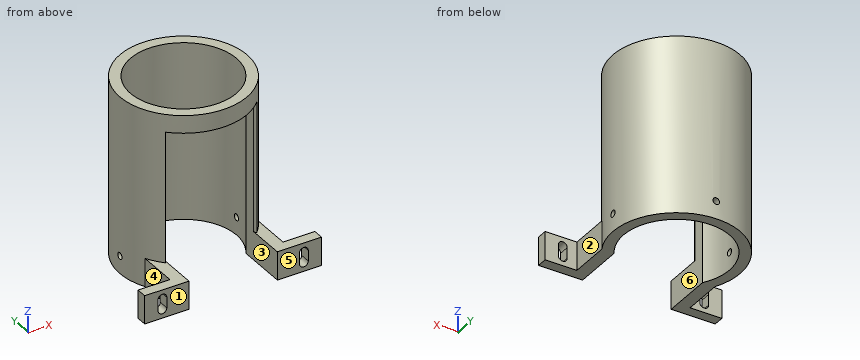
from build123d import *

# Parameters (mm, degrees)
SKETCH1_R                = 18
SKETCH1_R_2              = 15
BOSS_EXTRUDE1_DEPTH      = 50
SKETCH2_W                = 50
SKETCH2_H                = 8
BOSS_EXTRUDE2_DEPTH      = 3
BOSS_EXTRUDE5_REACH      = 69.315
BOSS_EXTRUDE5_END_RADIUS = 18
SKETCH9_W                = 32
SKETCH9_H                = 8
SKETCH4_W                = 37
SKETCH4_H                = 10
CUT_EXTRUDE1_DEPTH       = 75.204110398
CUT_EXTRUDE2_REACH       = 71.031
CUT_EXTRUDE2_END_RADIUS  = 15
SKETCH6_W                = 25
SKETCH6_H                = 45
FILLET1_R                = 1
CUT_EXTRUDE3_REACH       = 62.26
CUT_EXTRUDE3_END_RADIUS  = 18
SKETCH7_R                = 0.925
CIRPATTERN1_START        = 14.971451916
CIRPATTERN1_OUTLINE_R    = 0.925
CIRPATTERN1_DEPTH        = 3.028548184
CIRPATTERN1_START_2      = 14.9714519
CIRPATTERN1_2_OUTLINE_R  = 0.925
CIRPATTERN1_2_DEPTH      = 3.028548184


# Read off the part's stored shape, not the designer's step: CirPattern1
with BuildPart() as part:
    # Sketch1 → Boss-Extrude1 (new body)
    with BuildSketch(Plane.XY):
        Circle(SKETCH1_R)
        Circle(SKETCH1_R_2, mode=Mode.SUBTRACT)
    extrude(amount=BOSS_EXTRUDE1_DEPTH)



with BuildPart() as body_2:
    # Sketch2 → Boss-Extrude2 (new body)
    with BuildSketch(Plane(origin=(0, -22.5, 0), x_dir=(1, 0, 0), z_dir=(0, 1, 0))):
        with Locations((0, -4)):
            Rectangle(SKETCH2_W, SKETCH2_H)
        with BuildLine():
            Line((21.25, -2.5), (21.25, -5.5))
            ThreePointArc((21.25, -5.5), (20, -6.75), (18.75, -5.5))
            Line((18.75, -5.5), (18.75, -2.5))
            ThreePointArc((18.75, -2.5), (20, -1.25), (21.25, -2.5))
        make_face(mode=Mode.SUBTRACT)
        with BuildLine():
            Line((-21.25, -2.5), (-21.25, -5.5))
            ThreePointArc((-21.25, -5.5), (-20, -6.75), (-18.75, -5.5))
            Line((-18.75, -5.5), (-18.75, -2.5))
            ThreePointArc((-18.75, -2.5), (-20, -1.25), (-21.25, -2.5))
        make_face(mode=Mode.SUBTRACT)
    extrude(amount=BOSS_EXTRUDE2_DEPTH)


with BuildPart() as part_1:
    add(part.part)

    add(body_2.part)  # Boss-Extrude5 merges body 2
    # Boss-Extrude5: up to this cylinder (the profile starts outside it)
    boss_extrude5_end = Plane(origin=(0, 0, 4), z_dir=(0, 0, -1)) * Cylinder(BOSS_EXTRUDE5_END_RADIUS, 175.63, mode=Mode.PRIVATE)
    # Sketch9 → Boss-Extrude5 (add, up to the surface)
    with BuildSketch(Plane(origin=(0, -19.5, 0), x_dir=(1, 0, 0), z_dir=(0, 1, 0)), mode=Mode.PRIVATE) as boss_extrude5_sk1:
        with Locations((0, -4)):
            Rectangle(SKETCH9_W, SKETCH9_H)
    boss_extrude5_tool1 = extrude(boss_extrude5_sk1.sketch, amount=BOSS_EXTRUDE5_REACH, mode=Mode.PRIVATE) - boss_extrude5_end
    add(boss_extrude5_tool1.solids().sort_by_distance((0, -19.5, 4))[0])

    # Sketch4 → Cut-Extrude1 (cut, through all)
    with BuildSketch(Plane.ZY.offset(25)):
        with Locations((26.5, -17.5)):
            Rectangle(SKETCH4_W, SKETCH4_H)
    extrude(amount=-CUT_EXTRUDE1_DEPTH, mode=Mode.SUBTRACT)

    # Cut-Extrude2: up to this cylinder (the profile starts outside it)
    cut_extrude2_end = Plane(origin=(0, 0, 22.5), z_dir=(0, 0, -1)) * Cylinder(CUT_EXTRUDE2_END_RADIUS, 173.062, mode=Mode.PRIVATE)
    # Sketch6 → Cut-Extrude2 (cut, up to the surface)
    with BuildSketch(Plane.XZ.offset(22.5), mode=Mode.PRIVATE) as cut_extrude2_sk1:
        with Locations((0, 22.5)):
            Rectangle(SKETCH6_W, SKETCH6_H)
    cut_extrude2_tool1 = extrude(cut_extrude2_sk1.sketch, amount=-CUT_EXTRUDE2_REACH, mode=Mode.PRIVATE) - cut_extrude2_end
    add(cut_extrude2_tool1.solids().sort_by_distance((0, -22.5, 22.5))[0], mode=Mode.SUBTRACT)

    # Fillet1
    # the kernel refuses this fillet: 1 mm, written as the material it takes off along each edge
    with BuildSketch(Plane(origin=(-12.5, -12.5, 8), x_dir=(-1.0, 1.3760033648058773e-12, 0), z_dir=(0, 0, 1)), Plane(origin=(12.5, -12.5, 45), x_dir=(1.0, 1.3602776120652602e-12, 0), z_dir=(0, 0, -1))) as fillet1_piece_1:
        with BuildLine():
            CenterArc((1, -0.836369457), FILLET1_R, 123.241294146, 56.758705854)
            Line((0, -0.836369457), (-0.02, -0.836369457))
            Line((-0.02, -0.836369457), (-0.02, 0))
            Line((-0.02, 0), (0, 0.02))
            ThreePointArc((0, 0.02), (0.225916923, 0.02), (0.440870524, 0.016727389))
            Line((0.440870524, 0.016727389), (0.451833847, 0))
        make_face()
    extrude(amount=37, mode=Mode.SUBTRACT)

    # Cut-Extrude3: up to this cylinder (the profile starts inside it)
    cut_extrude3_end = Plane(origin=(0, 0, 5), z_dir=(0, 0, -1)) * Cylinder(CUT_EXTRUDE3_END_RADIUS, 161.52, mode=Mode.PRIVATE)
    # Sketch7 → Cut-Extrude3 (cut, up to the surface)
    with BuildSketch(Plane(origin=(0, 0, 0), x_dir=(0, 0, -1), z_dir=(1, 0, 0)), mode=Mode.PRIVATE) as cut_extrude3_sk1:
        with Locations((-5, 0)):
            Circle(SKETCH7_R)
    cut_extrude3_tool1 = extrude(cut_extrude3_sk1.sketch, amount=-CUT_EXTRUDE3_REACH, mode=Mode.PRIVATE) & cut_extrude3_end
    add(cut_extrude3_tool1.solids().sort_by_distance((0, 0, 5))[0], mode=Mode.SUBTRACT)

    # CirPattern1 outline → CirPattern1 (cut)
    with BuildSketch(Plane.YZ.offset(CIRPATTERN1_START)):
        with Locations((0, 5)):
            Circle(CIRPATTERN1_OUTLINE_R)
    extrude(amount=CIRPATTERN1_DEPTH, mode=Mode.SUBTRACT)

    # CirPattern1 2 outline → CirPattern1 2 (cut)
    with BuildSketch(Plane(origin=(0, 0, 0), x_dir=(1, 0, 0), z_dir=(0, 1, 0)).offset(CIRPATTERN1_START_2)):
        with Locations((0, -5)):
            Circle(CIRPATTERN1_2_OUTLINE_R)
    extrude(amount=CIRPATTERN1_2_DEPTH, mode=Mode.SUBTRACT)


solid = part_1.part
Can you work these out from the model? Positions are in its coordinate system, mm. Face numbers are marked on the shaded views. A direction names the side the tool comes from. Coordinates: 2 decimals unless noted, no trailing zeros. Loops run counter-clockwise (first coordinate to the right, second up) from the corner with the lowest first, then second, coordinate; pieces in that order, holes last. Notation, with made-up numbers: (-21.75, 54) - (19.25, 54) arc R8 cw to (19.25, 67) - close; hole circle Ø6 at (33, -11). An arc over 180 degrees is marked (long way). Put each result on its own line as item: value. Start each with the question number.
Item 1: Suppose I cut it at C-C (x = -20). Please give me the cut outline in (y, z), and give its area (3 significant figures).
Item 2: If we mould it in two halves opening along Y, with no side actions, what happens to the marked faces 1, 2 and 3? For each: +Y half, -Y half, draft (parallel to the pull), parting line (faces both ways), or undercut.
Item 3: Suppose I cut it at D-D (z = 26.5). Please give me the cut outline in (x, y).
Item 4: Suppose I cut it at A-A (y = 0). Please give me the cut outline in (x, z) (3 decimals), and give its area (3 significant figures).
Item 5: Which directions (+Z, -Z, +X, -X, +Y, -Y) give clear straight access to the entire face, cutting with the end or side of a thin tool? Please do the marked faces 4, 5 and 6.
Item 6: If I drill on line 1 along X through (y, z) = (-10, 28); line 2 along X through (y, z) = (0, 28); line 3 along Z through (x, y) = (0, 16) (3 decimals), over which ranges is the centre line in solid material (lowest first)?
Item 7: For pin 1 (6 mm diameter, centred on y = -13, z = 39.5, fed in from +X); pin 2 (1.1 mm diameter, centred on x = 0, z = 5, fed in from +Y); pin 3 (1 mm diameter, centred on y = -0.5, z = 44.5, fed in from -X); pin 4 (15.5 mm diameter, centred on y = -17, z = 24.5, fed in from -X), each with a flat end and sliding along its axis, tell me the tip position at first contact or that it passes through.
Item 8: Suppose I cut it at B-B (x = 0). Please give me the cut outline in (y, z) (3 decimals).
Here are the results:
1. outline: (-22.5, 0) - (-19.5, 0) - (-19.5, 1.25) - (-22.5, 1.25) - close; (-22.5, 6.75) - (-19.5, 6.75) - (-19.5, 8) - (-22.5, 8) - close
1. area: 7.50 mm²
2. face 1: -Y half
2. face 2: undercut
2. face 3: draft
3. outline: (-12.95, -12.5) arc R1 ccw to (-12.5, -11.66) - (-12.5, -8.29) arc R15 cw (long way) to (12.5, -8.29) - (12.5, -11.66) arc R1 ccw to (12.95, -12.5) arc R18 ccw (long way) to start
4. outline: (-18, 0) - (-15, 0) - (-15, 4.075) - (-18, 4.075) - close; (-18, 5.925) - (-15, 5.925) - (-15, 50) - (-18, 50) - close; (15, 0) - (18, 0) - (18, 4.075) - (15, 4.075) - close; (15, 5.925) - (18, 5.925) - (18, 50) - (15, 50) - close
4. area: 289 mm²
5. face 4: +Z, -Z, -X
5. face 5: +Z, -Z, +X, -X, -Y
5. face 6: -Z, -Y
6. line 1: -14.97 to -12.5, 12.5 to 14.97
6. line 2: -18 to -15, 15 to 18
6. line 3: 0 to 4.075, 5.925 to 50
7. pin 1: x = 14.97
7. pin 2: through
7. pin 3: x = -18
7. pin 4: x = -15.44
8. outline: (-18, 45) - (-15, 45) - (-15, 50) - (-18, 50) - close; (15, 0) - (18, 0) - (18, 4.075) - (15, 4.075) - close; (15, 5.925) - (18, 5.925) - (18, 50) - (15, 50) - close
